Geometry check sheet. Reference: the model listing, model coordinates, mm. A direction names the side the tool comes from. Give positions to 0.01 mm unless a question says otherwise; leave off trailing zeros. Write each loop counter-clockwise with the first axis right and the second up, starting at its lowest first coordinate (ties: lowest second). Pieces come first, ordered by that corner, then holes. Notation, with made-up numbers: (-2.75, 35.5) - (53.25, 35.5) arc R12 ccw to (53.25, 48.5) - close; hole circle Ø2 at (47.5, -17.5). An arc over 180 degrees is marked (long way). Write item = value, one per line. Start each with the question number.
(1) Section check B-B, the plane x = 0. Enter the section's corners in (y, z), plus the area to 3 significant figures.
(2) Section check A-A, the plane z = -5. Give the number of separate pieces and of enclosed holes in the cut face, plus the area to 3 significant figures.
(3) Access from +Z, -Z, +X, -X, +Y, -Y to the whole of each face (thin tool, end or side, straight path). Record for faces 1 (the flat face through (-245.555, 217.271, -4.93)), 2 (the cylindrical face through (-249.193, 166.682, -4.93)), 3 (the flat face through (217.271, 245.555, -4.93)).
(4) Depth check by flat-ended pin: pin 1 Ø4 at (y, z) = (91.5, -8) entering from -X; pin 2 Ø13.5 at (x, y) = (231.58, 231.58) entering from -Z; pin 3 Ø5 at (x, y) = (-231.58, 231.58) entering from +Z; pin 4 Ø4 at (y, z) = (221.5, -4) entering from -X. Enter the tip coordinate at first touch or a pass-through.
(5) Draft check along Y on faces 4 (the cylindrical face through (6.21, 282.43, -4.93)), 5 (the cylindrical face through (-159.776, 239.375, -4.93)), 6 (the flat face through (46, 280, 0)), 7 (the flat face through (-216.945, 245.229, -4.93)). Enter one of: pulls with the +Y half, pulls with the -Y half, needs draft (parallel to the pull), parting line crosses it, or undercut.
(6) Thickness scan on L1, parallel to X at y = 7, z = -5; L2, parallel to X at y = 53, z = -7.25; L3, parallel to Y at x = -249, z = -0.5. Record the ranges inside material, lowest first.
(7) Section check C-C, the plane x = 270. Enter the section's corners in (y, z).
Autodesk Inventor part; units mm, degrees
ref_plane "YZ Plane" through (0, 0, 0) normal (1, 0, 0) x (0, 1, 0)
ref_plane "XZ Plane" through (0, 0, 0) normal (0, 1, 0) x (-1, 0, 0)
ref_plane "XY Plane" through (0, 0, 0) normal (0, 0, 1) x (1, 0, 0)
sketch "Sketch7" plane through (0, 0, 0) normal (0, 0, 1) x (1, 0, 0)
  circle A0 centre (-231.5775, 231.5775) radius 4.25
  line L0 (-231.5775, 203.2932) -> (-203.2932, 231.5775)
  line L1 (-203.2932, 231.5775) -> (-231.5775, 259.8617)
  line L2 (-231.5775, 259.8617) -> (-259.8617, 231.5775)
  line L3 (-259.8617, 231.5775) -> (-231.5775, 203.2932)
  line L4 (-231.5775, 203.2932) -> (-231.5775, 259.8617) construction
  line L5 (-203.2932, 231.5775) -> (-259.8617, 231.5775) construction
  line L6 (-231.5775, 203.2932) -> (-191.5775, 203.2932) construction
  arc A1 (289.9795, 47.2262) -> (285.9788, 67.3391) centre (0, 0) ccw construction
  arc A2 (295.9015, 48.1906) -> (291.8191, 68.7143) centre (0, 0) ccw
  arc A3 (284.0576, 46.2617) -> (280.1386, 65.9639) centre (0, 0) ccw
  arc A4 (284.0576, 46.2617) -> (295.9015, 48.1906) centre (289.9795, 47.2262) ccw
  arc A5 (291.8191, 68.7143) -> (280.1386, 65.9639) centre (285.9788, 67.3391) ccw
  line L7 (0, 0) -> (289.9795, 47.2262) construction
  line L8 (0, 0) -> (293.8, 0) construction
  line L9 (0, 0) -> (285.9788, 67.3391) construction
  circle A6 centre (0, 0) radius 307.5
  circle A7 centre (0, 0) radius 282.5
  line L10 (-203.2932, 231.5775) -> (-185.1143, 213.3986)
  line L11 (-231.5775, 203.2932) -> (-213.3986, 185.1143)
  line L12 (-307.5, 0) -> (0, 0)
  line L13 (0, 0) -> (307.5, 0)
  line L14 (-231.5775, -203.2932) -> (-259.8617, -231.5775)
  line L15 (-259.8617, -231.5775) -> (-231.5775, -259.8617)
  circle A8 centre (-231.5775, -231.5775) radius 4.25
  line L16 (-231.5775, -259.8617) -> (-203.2932, -231.5775)
  line L17 (-203.2932, -231.5775) -> (-231.5775, -203.2932)
  line L18 (-203.2932, -231.5775) -> (-185.1143, -213.3986)
  line L19 (-231.5775, -203.2932) -> (-213.3986, -185.1143)
  line L20 (203.2932, -231.5775) -> (231.5775, -259.8617)
  line L21 (231.5775, -259.8617) -> (259.8617, -231.5775)
  circle A9 centre (231.5775, -231.5775) radius 4.25
  line L22 (259.8617, -231.5775) -> (231.5775, -203.2932)
  line L23 (231.5775, -203.2932) -> (203.2932, -231.5775)
  line L24 (231.5775, -203.2932) -> (213.3986, -185.1143)
  line L25 (203.2932, -231.5775) -> (185.1143, -213.3986)
  line L26 (231.5775, 203.2932) -> (259.8617, 231.5775)
  line L27 (259.8617, 231.5775) -> (231.5775, 259.8617)
  circle A10 centre (231.5775, 231.5775) radius 4.25
  line L28 (231.5775, 259.8617) -> (203.2932, 231.5775)
  line L29 (203.2932, 231.5775) -> (231.5775, 203.2932)
  line L30 (203.2932, 231.5775) -> (185.1143, 213.3986)
  line L31 (231.5775, 203.2932) -> (213.3986, 185.1143)
  arc A11 (254.9356, 157.7589) -> (243.3099, 175.158) centre (0, 0) ccw
  arc A12 (243.3099, 175.158) -> (233.571, 168.1471) centre (238.4404, 171.6526) ccw
  arc A13 (244.7314, 151.4444) -> (233.571, 168.1471) centre (0, 0) ccw
  arc A14 (244.7314, 151.4444) -> (254.9356, 157.7589) centre (249.8335, 154.6017) ccw
  arc A15 (175.158, 243.3099) -> (157.7589, 254.9356) centre (0, 0) ccw
  arc A16 (157.7589, 254.9356) -> (151.4444, 244.7314) centre (154.6017, 249.8335) ccw
  arc A17 (168.1471, 233.571) -> (151.4444, 244.7314) centre (0, 0) ccw
  arc A18 (168.1471, 233.571) -> (175.158, 243.3099) centre (171.6526, 238.4404) ccw
  arc A19 (68.7143, 291.8191) -> (48.1906, 295.9015) centre (0, 0) ccw
  arc A20 (48.1906, 295.9015) -> (46.2617, 284.0576) centre (47.2262, 289.9795) ccw
  arc A21 (65.9639, 280.1386) -> (46.2617, 284.0576) centre (0, 0) ccw
  arc A22 (65.9639, 280.1386) -> (68.7143, 291.8191) centre (67.3391, 285.9788) ccw
  arc A23 (-48.1906, 295.9015) -> (-68.7143, 291.8191) centre (0, 0) ccw
  arc A24 (-68.7143, 291.8191) -> (-65.9639, 280.1386) centre (-67.3391, 285.9788) ccw
  arc A25 (-46.2617, 284.0576) -> (-65.9639, 280.1386) centre (0, 0) ccw
  arc A26 (-46.2617, 284.0576) -> (-48.1906, 295.9015) centre (-47.2262, 289.9795) ccw
  arc A27 (-157.7589, 254.9356) -> (-175.158, 243.3099) centre (0, 0) ccw
  arc A28 (-175.158, 243.3099) -> (-168.1471, 233.571) centre (-171.6526, 238.4404) ccw
  arc A29 (-151.4444, 244.7314) -> (-168.1471, 233.571) centre (0, 0) ccw
  arc A30 (-151.4444, 244.7314) -> (-157.7589, 254.9356) centre (-154.6017, 249.8335) ccw
  arc A31 (-243.3099, 175.158) -> (-254.9356, 157.7589) centre (0, 0) ccw
  arc A32 (-254.9356, 157.7589) -> (-244.7314, 151.4444) centre (-249.8335, 154.6017) ccw
  arc A33 (-233.571, 168.1471) -> (-244.7314, 151.4444) centre (0, 0) ccw
  arc A34 (-233.571, 168.1471) -> (-243.3099, 175.158) centre (-238.4404, 171.6526) ccw
  arc A35 (-291.8191, 68.7143) -> (-295.9015, 48.1906) centre (0, 0) ccw
  arc A36 (-295.9015, 48.1906) -> (-284.0576, 46.2617) centre (-289.9795, 47.2262) ccw
  arc A37 (-280.1386, 65.9639) -> (-284.0576, 46.2617) centre (0, 0) ccw
  arc A38 (-280.1386, 65.9639) -> (-291.8191, 68.7143) centre (-285.9788, 67.3391) ccw
  arc A39 (-295.9015, -48.1906) -> (-291.8191, -68.7143) centre (0, 0) ccw
  arc A40 (-291.8191, -68.7143) -> (-280.1386, -65.9639) centre (-285.9788, -67.3391) ccw
  arc A41 (-284.0576, -46.2617) -> (-280.1386, -65.9639) centre (0, 0) ccw
  arc A42 (-284.0576, -46.2617) -> (-295.9015, -48.1906) centre (-289.9795, -47.2262) ccw
  arc A43 (-254.9356, -157.7589) -> (-243.3099, -175.158) centre (0, 0) ccw
  arc A44 (-243.3099, -175.158) -> (-233.571, -168.1471) centre (-238.4404, -171.6526) ccw
  arc A45 (-244.7314, -151.4444) -> (-233.571, -168.1471) centre (0, 0) ccw
  arc A46 (-244.7314, -151.4444) -> (-254.9356, -157.7589) centre (-249.8335, -154.6017) ccw
  arc A47 (-175.158, -243.3099) -> (-157.7589, -254.9356) centre (0, 0) ccw
  arc A48 (-157.7589, -254.9356) -> (-151.4444, -244.7314) centre (-154.6017, -249.8335) ccw
  arc A49 (-168.1471, -233.571) -> (-151.4444, -244.7314) centre (0, 0) ccw
  arc A50 (-168.1471, -233.571) -> (-175.158, -243.3099) centre (-171.6526, -238.4404) ccw
  arc A51 (-68.7143, -291.8191) -> (-48.1906, -295.9015) centre (0, 0) ccw
  arc A52 (-48.1906, -295.9015) -> (-46.2617, -284.0576) centre (-47.2262, -289.9795) ccw
  arc A53 (-65.9639, -280.1386) -> (-46.2617, -284.0576) centre (0, 0) ccw
  arc A54 (-65.9639, -280.1386) -> (-68.7143, -291.8191) centre (-67.3391, -285.9788) ccw
  arc A55 (48.1906, -295.9015) -> (68.7143, -291.8191) centre (0, 0) ccw
  arc A56 (68.7143, -291.8191) -> (65.9639, -280.1386) centre (67.3391, -285.9788) ccw
  arc A57 (46.2617, -284.0576) -> (65.9639, -280.1386) centre (0, 0) ccw
  arc A58 (46.2617, -284.0576) -> (48.1906, -295.9015) centre (47.2262, -289.9795) ccw
  arc A59 (157.7589, -254.9356) -> (175.158, -243.3099) centre (0, 0) ccw
  arc A60 (175.158, -243.3099) -> (168.1471, -233.571) centre (171.6526, -238.4404) ccw
  arc A61 (151.4444, -244.7314) -> (168.1471, -233.571) centre (0, 0) ccw
  arc A62 (151.4444, -244.7314) -> (157.7589, -254.9356) centre (154.6017, -249.8335) ccw
  arc A63 (243.3099, -175.158) -> (254.9356, -157.7589) centre (0, 0) ccw
  arc A64 (254.9356, -157.7589) -> (244.7314, -151.4444) centre (249.8335, -154.6017) ccw
  arc A65 (233.571, -168.1471) -> (244.7314, -151.4444) centre (0, 0) ccw
  arc A66 (233.571, -168.1471) -> (243.3099, -175.158) centre (238.4404, -171.6526) ccw
  arc A67 (291.8191, -68.7143) -> (295.9015, -48.1906) centre (0, 0) ccw
  arc A68 (295.9015, -48.1906) -> (284.0576, -46.2617) centre (289.9795, -47.2262) ccw
  arc A69 (280.1386, -65.9639) -> (284.0576, -46.2617) centre (0, 0) ccw
  arc A70 (280.1386, -65.9639) -> (291.8191, -68.7143) centre (285.9788, -67.3391) ccw
  point P0 (-202.8328, 231.1171)
  point P1 (-231.1171, 202.8328)
  point P2 (-282.5, 0)
  point P3 (282.5, 0)
  point P4 (231.1171, 202.8328)
  point P5 (202.8328, 231.1171)
  dimension "d131" = 8.5
  dimension "d132" = 231.5775
  dimension "d133" = 231.5775
  dimension "d135" = 45
  dimension "d137" = 40
  dimension "d138" = 40
  dimension "d144" = 293.8
  dimension "d145" = 9.25
  dimension "d146" = 4
  dimension "d147" = 12
  dimension "d148" = 615
  dimension "d149" = 565
  dimension "d152" = 360
  dimension "d156" = 360
extrude "Extrusion11" add sketch "Sketch7" against normal blind 10 contours L3 L2 L1 L0 | L0 A6 L11 | L0 L10 A6 | A6 L10 A7 L11 | L11 A7 L12 A6 | A6 L30 A7 L10 | L30 L29 A6 | A6 L31 A7 L30 | L29 L31 A6 | L29 L28 L27 L26 | A6 L13 A7 L31
sketch "Sketch8" plane through (-307.5, 0, 0) normal (0, -1, 0) x (1, 0, 0)
  line L0 (25, 0) -> (590, 0)
  line L1 (25, 0) -> (-15, 0)
  line L2 (-15, 0) -> (-15, -10)
  line L3 (-15, -10) -> (25, -10)
  line L4 (25, -10) -> (25, 0)
  circle A0 centre (-7.5, -5) radius 2.6
  line L5 (590, 0) -> (630, 0)
  line L6 (630, 0) -> (630, -10)
  line L7 (630, -10) -> (590, -10)
  line L8 (590, -10) -> (590, 0)
  circle A1 centre (622.5, -5) radius 2.6
  dimension "d160" = 40
  dimension "d161" = 10
  dimension "d162" = 5.2
  dimension "d163" = 5
  dimension "d164" = 7.5
  dimension "d165" = 40
  dimension "d166" = 10
  dimension "d167" = 5.2
  dimension "d168" = 7.5
  dimension "d169" = 5
extrude "Extrusion12" add sketch "Sketch8" against normal blind 10 contours L5 L6 L7 L8 | L4 L3 L2 L1 | A0 | A1
fillet "Fillet4" radius 4 8 edges at (-231.1171, 202.8328, -5) (-259.8617, 231.5775, -5) (-202.8328, 231.1171, -5) (-231.5775, 259.8617, -5) (231.5775, 259.8617, -5) (259.8617, 231.5775, -5) (202.8328, 231.1171, -5) (231.1171, 202.8328, -5)
hole "Hole6" at (-315, 0, -5) at (315, 0, -5) direction (0, 1, 0) diameter 5.2 end through all
equation "\"bar_screw_hole_diam\" = 8.5"
equation "\"foot_length\" = 15"
equation "\"tube_rim_diam\" = 605"
equation "\"tube_inner_diam\" = 541"
equation "\"tube_outer_diam\" = 561"
equation "\"ring_delta\" = 2"
equation "\"bar_delta\" = 5"
equation "\"bar_circle_diam\" = 655"
equation "\"ring_inner_diam\" = 565"
equation "\"ring_outer_diam\" = 615"
equation "\"slot_angle\" = 9.25deg"
equation "\"slot_diam\" = 12"
equation "\"slots_circle_diam\" = 587.6"
equation "\"foot_screw_diam\" = 5.2"
equation "\"bar_fillet\" = 4"
properties part number "half_ring_1" material "Aluminum 6061"
Model answer:
q1.outline = (282.5, -10) - (307.5, -10) - (307.5, 0) - (282.5, 0) - close
q1.area = 250 mm²
q2.separate_pieces = 3
q2.enclosed_holes = 10
q2.area = 23,600 mm²
q3.face_1 = +Z, -Z, -X
q3.face_2 = +Z, -Z
q3.face_3 = +Z, -Z, +Y
q4.pin_1 = -294.19
q4.pin_2 = -10
q4.pin_3 = through
q4.pin_4 = -251.78
q5.face_4 = pulls with the -Y half
q5.face_5 = undercut
q5.face_6 = needs draft
q5.face_7 = pulls with the +Y half
q6.L1 = -322.5 to -317.6, -312.4 to -282.41, 282.41 to 312.4, 317.6 to 322.5
q6.L2 = -302.9 to -295.08, -282.88 to -277.48, 277.48 to 282.88, 295.08 to 302.9
q6.L3 = 133.44 to 148.66, 166.97 to 180.43, 220.72 to 242.44
q7.outline = (83.1, -10) - (147.16, -10) - (147.16, 0) - (83.1, 0) - close
